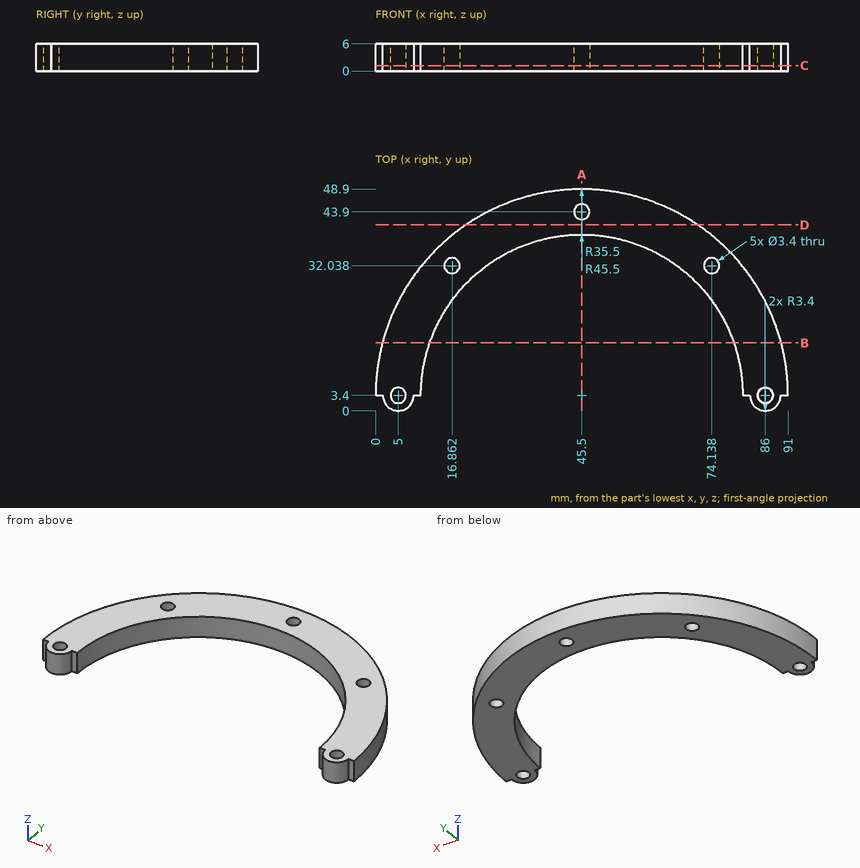
Can you work these out from the drawing? Everything is in mm from the part's minimum corner. Coordinates: 2 decimals unless noted, no trailing zeros. Order: outer loops, then holes, each group sorted by start corner. A loop starts at its lowest first (then second) coordinate and runs counter-clockwise, first axis right, second up. Notation, with made-up numbers: M 85.25,-10.75 L 92.25,-10.75 A18 ccw 92.25,9.25 Z; hole C 31.25,-3.75 d3. An arc over 180 degrees is marked long. Answer as CSV lines item,"result". Start each with the question number.
1. I want a section at A-A, the plane x = 45.5. Write out the boundary of the cut face in (y, z).
2. I want a section at C-C, the plane z = 1.25. Write out the boundary of the cut face in (x, y).
3. I want a section at D-D, the plane y = 41. Write out the boundary of the cut face in (x, z).
4. I want a section at B-B, the plane y = 15. Write out the boundary of the cut face in (x, z), and give its area (3 significant figures).
5. For pin 1 (0.8 mm diameter, centred on x = 9, z = 1.5, fed in from -Y); pin 2 (1.8 mm diameter, centred on x = 90, z = 3, fed in from -Y), each with a flat end and sliding along its axis, tell me the tip position at first contact or that it passes through.
6. I need wall thicknesses on line 1 (X direction, y = 15, z = 0.9); line 2 (X direction, y = 27, z = 5.05); line 3 (Y direction, x = 17.5, z = 5.05) (1 decimal). Which ranges of each line are inside material? Lowest first, please. Write a range as [from, to].
Recorded:
1,outline,"M 38.9,0 L 42.2,0 L 42.2,6 L 38.9,6 Z; M 45.6,0 L 48.9,0 L 48.9,6 L 45.6,6 Z"
2,outline,"M 0,3.4 L 1.6,3.4 A3.4 ccw 8.4,3.4 L 10,3.4 A35.5 cw 81,3.4 L 82.6,3.4 A3.4 ccw 89.4,3.4 L 91,3.4 A45.5 ccw Z; hole C 5,3.4 d3.4; hole C 16.86,32.04 d3.4; hole C 45.5,43.9 d3.4; hole C 74.14,32.04 d3.4; hole C 86,3.4 d3.4"
3,outline,"M 19.88,0 L 71.12,0 L 71.12,6 L 19.88,6 Z"
4,outline,"M 1.5,0 L 11.95,0 L 11.95,6 L 1.5,6 Z; M 79.05,0 L 89.5,0 L 89.5,6 L 79.05,6 Z"
4,area,"125 mm2"
5,pin 1,"stops at y = 3.4"
5,pin 2,"stops at y = 2"
6,line 1,"x = [1.5, 11.95], [79.05, 89.5]"
6,line 2,"x = [6.6, 18.98], [72.02, 84.4]"
6,line 3,"y = [25.2, 30.5], [33.6, 39.3]"
